Model file for the job. Use its own axes, mm. Face numbers are marked on the shaded views. A direction names the side the tool comes from. Give positions to 0.01 mm unless a question says otherwise; leave off trailing zeros. Loops run counter-clockwise (first coordinate to the right, second up) from the corner with the lowest first, then second, coordinate; pieces in that order, holes last. Notation, with made-up numbers: (61, 72.25) - (94, 72.25) arc R16 cw to (94, 78.25) - close; hole circle Ø5 at (-13, 86.25). An arc over 180 degrees is marked (long way). Use a Markdown table: item, result.
from build123d import *


with BuildPart() as part:
    # Sketch1 → Revolve1 (revolve)
    with BuildSketch(Plane(origin=(0, 0, 0), x_dir=(1, 0, 0), z_dir=(0, 1, 0)), mode=Mode.PRIVATE) as revolve1_sk:
        Polygon((0, 0), (-36, 0), (-36, 12.5), (-30, 12.5), (-30, 7.5), (30, 7.5), (30, 12.5), (36, 12.5), (36, 0), align=None)
    revolve(revolve1_sk.sketch.rotate(Axis((-414.016836438, 0, 0), (1, 0, 0)), 180), axis=Axis((-414.016836438, 0, 0), (1, 0, 0)))


solid = part.part
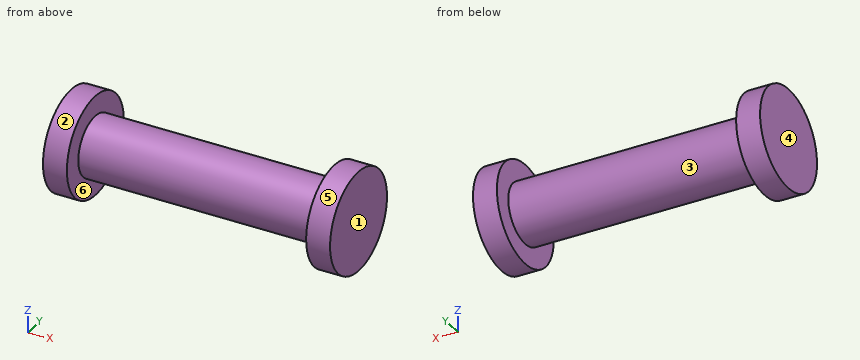
(1) Slice it at B-B, the plane y = 0. Write the cut outline in (x, z), plus the area to 3 significant figures.
Computed:
| item | result |
|---|---|
| outline | (-36, -12.5) - (-30, -12.5) - (-30, -7.5) - (30, -7.5) - (30, -12.5) - (36, -12.5) - (36, 12.5) - (30, 12.5) - (30, 7.5) - (-30, 7.5) - (-30, 12.5) - (-36, 12.5) - close |
| area | 1,200 mm² |
(2) Drill centre lines: probe 1 along X at (y, z) = (-8, -7); probe 2 along Y at (x, z) = (-15, 0.25); probe 3 along Y at (x, z) = (-24, -5.75). Where is each one in solid material? Low to high. Write a range as [from, to].
Computed:
| item | result |
|---|---|
| probe 1 | [-36, -30], [30, 36] |
| probe 2 | [-7.5, 7.5] |
| probe 3 | [-4.82, 4.82] |
(3) Slice it at A-A, the plane z = -10. Write the cut outline in (x, y).
Computed:
| item | result |
|---|---|
| outline | (-36, -7.5) - (-30, -7.5) - (-30, 7.5) - (-36, 7.5) - close; (30, -7.5) - (36, -7.5) - (36, 7.5) - (30, 7.5) - close |
(4) Slice it at D-D, the plane y = 10.75. Write the cut outline in (x, z).
Computed:
| item | result |
|---|---|
| outline | (-36, -6.38) - (-30, -6.38) - (-30, 6.38) - (-36, 6.38) - close; (30, -6.38) - (36, -6.38) - (36, 6.38) - (30, 6.38) - close |
(5) Pin check, flat tips, straight feed: P1, Ø3, axis at x = -18.5, y = -4, coming from the +Z side; P2, Ø12, axis at x = 22, z = -9, coming from the +Y side; P3, Ø5, axis at x = 0.5, y = 1.5, coming from the -Z side. Stop position of each tip, or through.
Computed:
| item | result |
|---|---|
| P1 | z = 7.07 |
| P2 | y = 6.87 |
| P3 | z = -7.5 |
(6) 3-axis set-ups, long thin cutter, end or side, ignore diameter. For the marked faces 5 and 6: which of +Z, -Z, +X, -X, +Y, -Y reach the whole face in a straight line?
Computed:
| item | result |
|---|---|
| face 5 | +X, -X |
| face 6 | none |
(7) Mould opens along X. For the marked faces 1, 2, 3 and 4 say: pulls with the +X half, pulls with the -X half, needs draft (parallel to the pull), parting line crosses it, or undercut.
Computed:
| item | result |
|---|---|
| face 1 | pulls with the +X half |
| face 2 | needs draft |
| face 3 | undercut |
| face 4 | pulls with the -X half |
